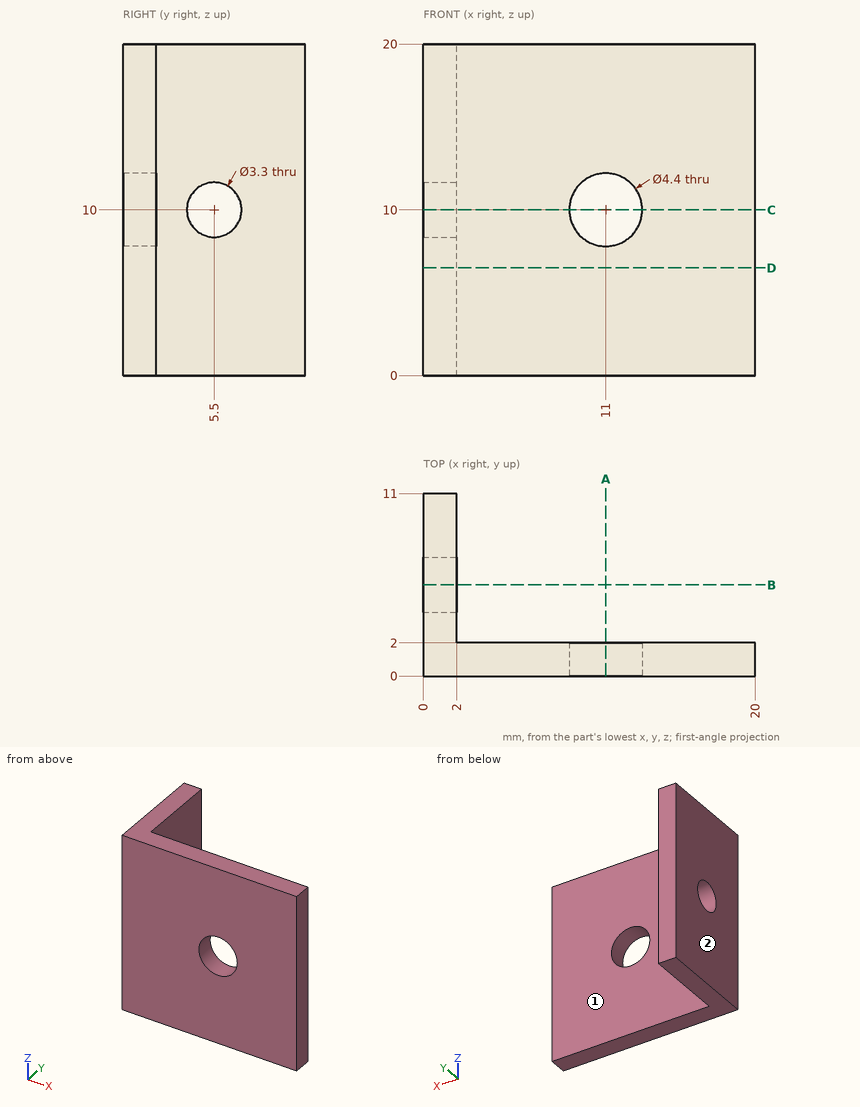
Can you work these out from the drawing? Everything is in mm from the part's minimum corner. A direction names the side the tool comes from. Round coordinates to 2 decimals unless told otherwise and drop trailing zeros. Loops run counter-clockwise (first coordinate to the right, second up) from the corner with the lowest first, then second, coordinate; pieces in that order, holes last. Notation, with made-up numbers: (31, 23) - (56, 23) arc R30 ccw to (56, 55) - close; hole circle Ø1 at (40.25, 16). An arc over 180 degrees is marked (long way). Answer in a Markdown table with one row per item. Add a question column.
(1) For the marked faces 1 and 2, which set-ups out of +Z, -Z, +X, -X, +Y, -Y let a thin tool reach every point of the face, with its end or its side?
(2) If we section it at A-A (x = 11): Please give me the cut outline in (y, z).
(3) If we section it at B-B (y = 5.5): Please give me the cut outline in (x, z).
(4) I need wall thicknesses on line 1 along Z through (x, y) = (11, 1.5); line 2 along Z through (x, y) = (1.4, 5.5); line 3 along Y through (x, z) = (18.75, 12.5). Which ranges of each line are inside material? Lowest first, please.
(5) I'm going to push flat-ended pins straight in: pin 1 (5.5 mm diameter, centred on y = 5.5, z = 10, fed in from +X); pin 2 (2 mm diameter, centred on x = 7, z = 17, fed in from +Y). Where does each tip first touch, or does it pass through?
(6) If we section it at D-D (z = 6.5): Please give me the cut outline in (x, y).
(7) If we section it at C-C (z = 10): Please give me the cut outline in (x, y), plus the area to 3 significant figures.
Model answer:
| question | item | result |
|---|---|---|
| 1 | face 1 | +Z, -Z, +X, +Y |
| 1 | face 2 | +Z, -Z, -X, +Y, -Y |
| 2 | outline | (0, 0) - (2, 0) - (2, 7.8) - (0, 7.8) - close; (0, 12.2) - (2, 12.2) - (2, 20) - (0, 20) - close |
| 3 | outline | (0, 0) - (2, 0) - (2, 8.35) - (0, 8.35) - close; (0, 11.65) - (2, 11.65) - (2, 20) - (0, 20) - close |
| 4 | line 1 | z = 0 to 7.8, 12.2 to 20 |
| 4 | line 2 | z = 0 to 8.35, 11.65 to 20 |
| 4 | line 3 | y = 0 to 2 |
| 5 | pin 1 | stops at x = 2 |
| 5 | pin 2 | stops at y = 2 |
| 6 | outline | (0, 0) - (20, 0) - (20, 2) - (2, 2) - (2, 11) - (0, 11) - close |
| 7 | outline | (0, 0) - (8.8, 0) - (8.8, 2) - (2, 2) - (2, 3.85) - (0, 3.85) - close; (0, 7.15) - (2, 7.15) - (2, 11) - (0, 11) - close; (13.2, 0) - (20, 0) - (20, 2) - (13.2, 2) - close |
| 7 | area | 42.6 mm² |
